Geometry check sheet. Reference: drawing and pictorial views, mm from the part's lowest x, y, z. Give positions to 0.01 mm unless a question says otherwise; leave off trailing zeros. Write each loop counter-clockwise with the first axis right and the second up, starting at its lowest first coordinate (ties: lowest second). Pieces come first, ordered by that corner, then holes.
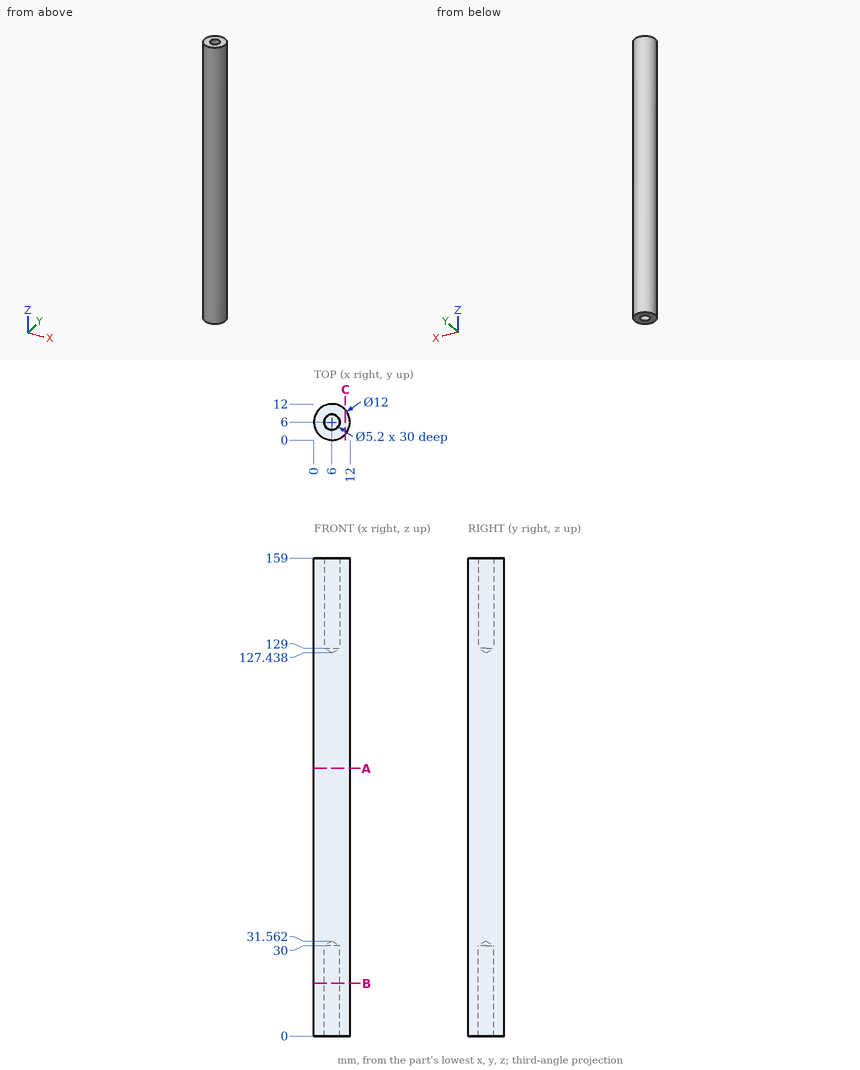
Item 1: Sectioned sample at B-B on z = 17.5. Record the cut outline in (x, y).
Answer key:
outline: circle Ø12 at (6, 6); hole circle Ø5.2 at (6, 6)
Item 2: Sectioned sample at A-A on z = 89. Record the cut outline in (x, y).
Answer key:
outline: circle Ø12 at (6, 6)
Item 3: Scan lines: line 1 along Y through (x, z) = (6, 142.5); line 2 along Y through (x, z) = (5.75, 31) (1 decimal); line 3 along X through (y, z) = (6.75, 134). Record each from-to range of solid material in increasing order.
Answer key:
line 1: y = 0 to 3.4, 8.6 to 12
line 2: y = 0 to 5.1, 6.9 to 12
line 3: x = 0.05 to 3.51, 8.49 to 11.95
Item 4: Sectioned sample at C-C on x = 10.5. Record the cut outline in (y, z).
Answer key:
outline: (2.03, 0) - (9.97, 0) - (9.97, 159) - (2.03, 159) - close
Item 5: Depth check by flat-ended pin: pin 1 (4 mm diameter, centred on x = 6, y = 6, fed in from +Z); pin 2 (1.5 mm diameter, centred on x = 9, z = 79.5, fed in from -Y); pin 3 (1 mm diameter, centred on y = 10.5, z = 79.5, fed in from +X). Enter the tip coordinate at first touch or a pass-through.
Answer key:
pin 1: stops at z = 128.64
pin 2: stops at y = 0.44
pin 3: stops at x = 10.47
